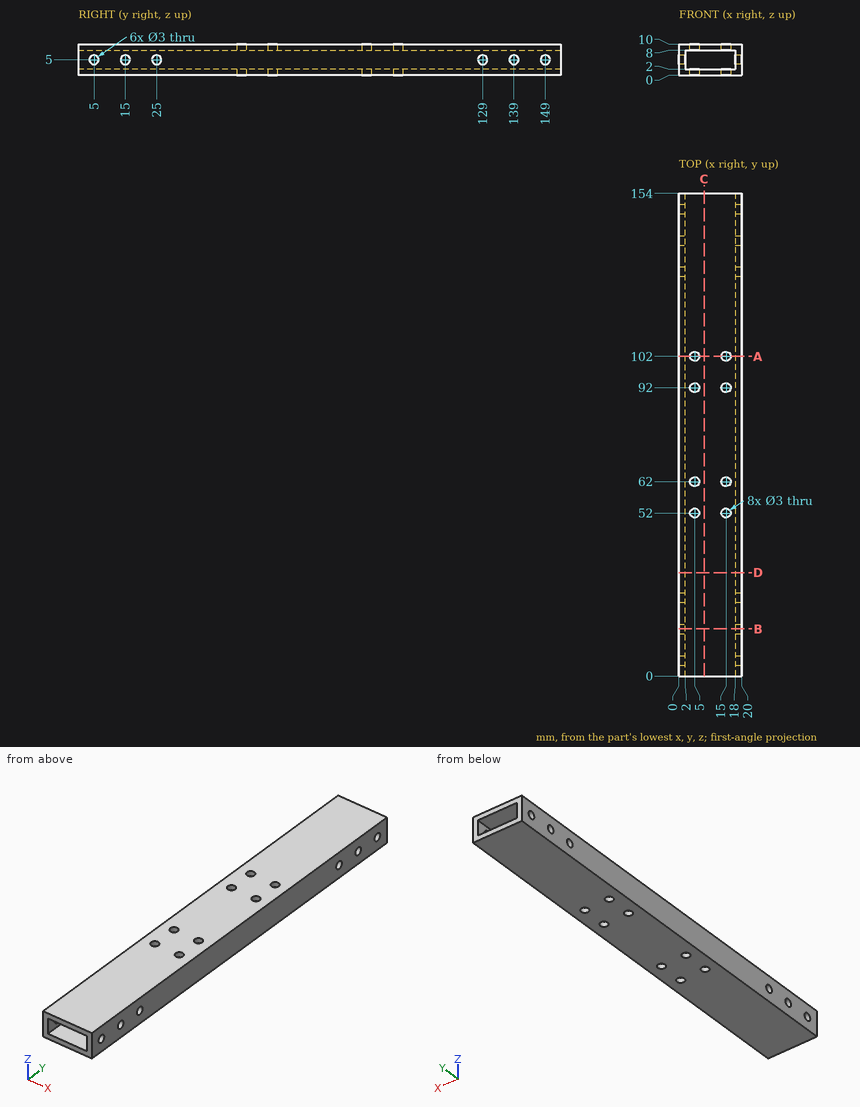
Could you check a few things on this drawing? It's one solid part, dimensions in mm from its lowest x, y, z. Round coordinates to 2 decimals unless told otherwise and drop trailing zeros. Order: outer loops, then holes, each group sorted by start corner. A loop starts at its lowest first (then second) coordinate and runs counter-clockwise, first axis right, second up. Notation, with made-up numbers: M 13,-38 L 58,-38 A18 cw 58,-21 Z; hole C -0.5,27.25 d3. An arc over 180 degrees is marked long. One line per item, written item: value.
(1) Imagine slicing it at B-B (y = 15). Write out the boundary of the cut face in (x, z), and give its area (3 significant figures).
Ans:
outline: M 0,0 L 20,0 L 20,3.5 L 18,3.5 L 18,2 L 2,2 L 2,3.5 L 0,3.5 Z; M 0,6.5 L 2,6.5 L 2,8 L 18,8 L 18,6.5 L 20,6.5 L 20,10 L 0,10 Z
area: 92.0 mm^2
(2) Imagine slicing it at C-C (x = 8). Write out the boundary of the cut face in (y, z), and give its area (3 significant figures).
Ans:
outline: M 0,0 L 154,0 L 154,2 L 0,2 Z; M 0,8 L 154,8 L 154,10 L 0,10 Z
area: 616 mm^2
(3) I need wall thicknesses on line 1 along X through (y, z) = (92, 1.4); line 2 along Y through (x, z) = (5.25, 8.5); line 3 along Z through (x, y) = (12.75, 110). Which ranges of each line are inside material? Lowest first, please. Write a range as from..to.
Ans:
line 1: x = 0..3.5, 6.5..13.5, 16.5..20
line 2: y = 0..50.52, 53.48..60.52, 63.48..90.52, 93.48..100.52, 103.48..154
line 3: z = 0..2, 8..10
(4) Imagine slicing it at A-A (y = 102). Write out the boundary of the cut face in (x, z), and give its area (3 significant figures).
Ans:
outline: M 0,0 L 3.5,0 L 3.5,2 L 2,2 L 2,8 L 3.5,8 L 3.5,10 L 0,10 Z; M 6.5,0 L 13.5,0 L 13.5,2 L 6.5,2 Z; M 6.5,8 L 13.5,8 L 13.5,10 L 6.5,10 Z; M 16.5,0 L 20,0 L 20,10 L 16.5,10 L 16.5,8 L 18,8 L 18,2 L 16.5,2 Z
area: 80.0 mm^2
(5) Imagine slicing it at D-D (y = 33). Write out the boundary of the cut face in (x, z), and give its area (3 significant figures).
Ans:
outline: M 0,0 L 20,0 L 20,10 L 0,10 Z; hole M 2,2 L 18,2 L 18,8 L 2,8 Z
area: 104 mm^2
(6) I'm going to push flat-ended pins straight in: P1, Ø5, axis at x = 15.5, y = 86, coming from the -Z side; P2, Ø1.8, axis at y = 15, z = 5, coming from the +X side. Where does each tip first touch, or does it pass through?
Ans:
P1: stops at z = 0
P2: passes through
